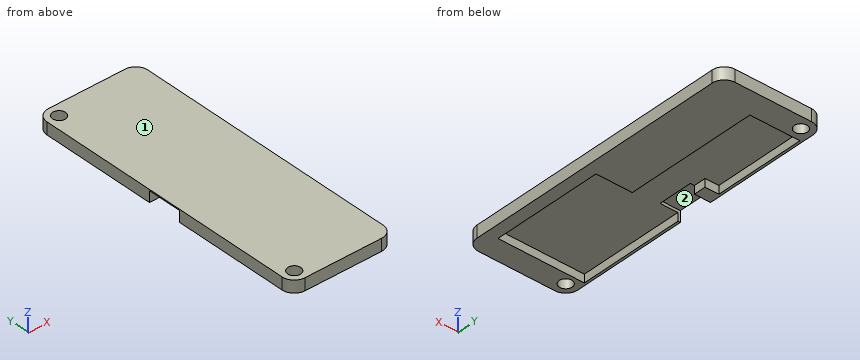
from build123d import *

# Parameters (mm, degrees)
SKETCH1_R           = 1.6
BOSS_EXTRUDE1_DEPTH = 3
CUT_EXTRUDE1_DEPTH  = 2
SKETCH3_W           = 5
SKETCH3_H           = 8.5
CUT_EXTRUDE2_DEPTH  = 2.7
SKETCH4_W           = 4
SKETCH4_H           = 3
BOSS_EXTRUDE2_DEPTH = 2
FILLET1_R           = 3


with BuildPart() as part:
    # Sketch1 → Boss-Extrude1 (new body)
    with BuildSketch(Plane.XY):
        with BuildLine():
            Line((0, 36), (0, -36))
            Line((0, -36), (-22, -36))
            ThreePointArc((-22, -36), (-24.121320344, -35.121320344), (-25, -33))
            Line((-25, -33), (-25, 33))
            ThreePointArc((-25, 33), (-24.121320344, 35.121320344), (-22, 36))
            Line((-22, 36), (0, 36))
        make_face()
        with Locations((-22, 33)):
            Circle(SKETCH1_R, mode=Mode.SUBTRACT)
        with Locations((-22, -33)):
            Circle(SKETCH1_R, mode=Mode.SUBTRACT)
    extrude(amount=BOSS_EXTRUDE1_DEPTH)

    # Sketch2 → Cut-Extrude1 (cut)
    with BuildSketch(Plane(origin=(0, 0, 0), x_dir=(-1, 0, 0), z_dir=(0, 0, -1))):
        Polygon((24.4, 30), (12, 30), (12, -3), (3, -3), (3, -30.5), (24.4, -30.5), align=None)
    extrude(amount=-CUT_EXTRUDE1_DEPTH, mode=Mode.SUBTRACT)

    # Sketch3 → Cut-Extrude2 (cut)
    with BuildSketch(Plane(origin=(0, 0, 0), x_dir=(-1, 0, 0), z_dir=(0, 0, -1))):
        with Locations((22.5, 0)):
            Rectangle(SKETCH3_W, SKETCH3_H)
    extrude(amount=-CUT_EXTRUDE2_DEPTH, mode=Mode.SUBTRACT)

    # Sketch4 → Boss-Extrude2 (add)
    with BuildSketch(Plane(origin=(0, 0, 0), x_dir=(-1, 0, 0), z_dir=(0, 0, -1))):
        with Locations((23, 5.75)):
            Rectangle(SKETCH4_W, SKETCH4_H)
    extrude(amount=-BOSS_EXTRUDE2_DEPTH)

    # Fillet1
    fillet1_edges = [part.edges().sort_by_distance(p)[0] for p in [
        (0, 36, 1.5),
        (0, -36, 1.5),
    ]]
    fillet(fillet1_edges, radius=FILLET1_R)


solid = part.part
Verification items for the finished model (mm, model axes). Face numbers are marked on the shaded views. Give positions to 0.01 mm unless a question says otherwise; leave off trailing zeros. Write each loop counter-clockwise with the first axis right and the second up, starting at its lowest first coordinate (ties: lowest second). Pieces come first, ordered by that corner, then holes. Notation, with made-up numbers: M 56.25,57.5 L 96.25,57.5 A19 ccw 96.25,64.5 Z; hole C 74.5,6.25 d2. An arc over 180 degrees is marked long. Put each result on its own line as item: value. Start each with the question number.
1. Section check C-C (x = -3.75). Record the cut outline in (y, z), and give its area (3 significant figures).
2. Scan lines: line 1 along Y through (x, z) = (-22, 1.4); line 2 along Y through (x, z) = (-10.75, 0.9); line 3 along Y through (x, z) = (-19, 1.55). Record each from-to range of solid material in increasing order. Write a range as [from, to].
3. Section check A-A (z = 0.5). Record the cut outline in (x, y), and give its area (3 significant figures).
4. Go/stop test with flat-tipped pins: pin 1 Ø2.5 at (x, y) = (-22.5, 0) entering from -Z; pin 2 Ø1.9 at (x, y) = (-22, 33) entering from +Z; pin 3 Ø2 at (x, y) = (-20.5, 1) entering from -Z; pin 4 Ø1.4 at (x, z) = (-23, 1.5) entering from +Y. Record where each tip stops, or that it passes through.
5. Draft check along Y on the marked faces 1 and 2. Enter one of: +Y half, -Y half, draft (parallel to the pull), parting line (faces both ways), or undercut.
6. Section check B-B (y = -17). Record the cut outline in (x, z).
Answer list:
1. outline: M -36,0 L -30.5,0 L -30.5,2 L -3,2 L -3,0 L 36,0 L 36,3 L -36,3 Z
1. area: 161 mm2
2. line 1: [-36, -34.6], [-31.4, -30.5], [4.25, 7.25], [30, 31.4], [34.6, 36]
2. line 2: [-36, -30.5], [-3, 36]
2. line 3: [-36, -30.5], [30, 36]
3. outline: M -25,-33 A3 ccw -22,-36 L -3,-36 A3 ccw 0,-33 L 0,33 A3 ccw -3,36 L -22,36 A3 ccw -25,33 L -25,4.25 L -21,4.25 L -21,7.25 L -24.4,7.25 L -24.4,30 L -12,30 L -12,-3 L -3,-3 L -3,-30.5 L -24.4,-30.5 L -24.4,-4.25 L -25,-4.25 Z; hole C -22,-33 d3.2; hole C -22,33 d3.2
3. area: 784 mm2
4. pin 1: z = 2.7
4. pin 2: through
4. pin 3: z = 2
4. pin 4: y = 35.98
5. face 1: draft
5. face 2: undercut
6. outline: M -25,0 L -24.4,0 L -24.4,2 L -3,2 L -3,0 L 0,0 L 0,3 L -25,3 Z
